Source: CAD feature listing. Evaluate the final solid. Frame: model axes, mm. A direction names the side the tool comes from. Round coordinates to 2 decimals unless told otherwise and drop trailing zeros.
Autodesk Fusion 360 part; units mm, degrees
sketch "Sketch1" plane through (0, 0, 0) normal (0, 1, 0) x (1, 0, 0)
  line L0 (20, -40) -> (-20, 40) construction
  line L1 (-20, -40) -> (20, 40) construction
  line L2 (5, 29) -> (-5, 29)
  line L3 (-5, 29) -> (-5, 39)
  line L4 (5, 39) -> (5, 29)
  line L5 (5, 29) -> (-5, 39) construction
  line L6 (-5, 29) -> (5, 39) construction
  line L7 (-4, 39) -> (-4, 40)
  line L8 (4, 39) -> (4, 40)
  line L9 (-19, 25) -> (-9, 25)
  line L10 (-9, 25) -> (-9, 15)
  line L11 (-9, 15) -> (-19, 15)
  line L12 (19, 25) -> (9, 25)
  line L13 (9, 25) -> (9, 15)
  line L14 (9, 15) -> (19, 15)
  line L15 (-20, 16) -> (-19, 16)
  line L16 (-19, 24) -> (-20, 24)
  line L17 (19, 16) -> (20, 16)
  line L18 (20, 24) -> (19, 24)
  line L19 (-20, 24) -> (-20, 40)
  line L20 (-19, 15) -> (-19, 16)
  line L21 (-19, 24) -> (-19, 25)
  line L22 (19, 15) -> (19, 16)
  line L23 (19, 24) -> (19, 25)
  line L24 (-20, 40) -> (-4, 40)
  line L25 (4, 40) -> (20, 40)
  line L26 (-5, 39) -> (-4, 39)
  line L27 (4, 39) -> (5, 39)
  line L28 (20, 40) -> (20, 24)
  line L29 (1.75, 0) -> (22.5, 0)
  line L30 (-19, -24) -> (-20, -24)
  line L31 (-19, -24) -> (-19, -25)
  line L32 (-19, -25) -> (-9, -25)
  line L33 (-20, -16) -> (-19, -16)
  line L34 (-19, -15) -> (-19, -16)
  line L35 (-9, -15) -> (-19, -15)
  line L36 (-9, -25) -> (-9, -15)
  line L37 (-4, -39) -> (-4, -40)
  line L38 (-5, -39) -> (-4, -39)
  line L39 (-5, -29) -> (-5, -39)
  line L40 (5, -29) -> (-5, -29)
  line L41 (5, -39) -> (5, -29)
  line L42 (4, -39) -> (5, -39)
  line L43 (4, -39) -> (4, -40)
  line L44 (20, -24) -> (19, -24)
  line L45 (19, -24) -> (19, -25)
  line L46 (19, -25) -> (9, -25)
  line L47 (9, -25) -> (9, -15)
  line L48 (9, -15) -> (19, -15)
  line L49 (19, -15) -> (19, -16)
  line L50 (19, -16) -> (20, -16)
  line L51 (-20, -40) -> (-20, -24)
  line L52 (-20, -16) -> (-20, 16)
  line L53 (20, 16) -> (20, -16)
  line L54 (20, -24) -> (20, -40)
  line L55 (20, -40) -> (4, -40)
  line L56 (-4, -40) -> (-20, -40)
  point P0 (0, 34)
  dimension "d20" = 40
  dimension "d21" = 80
  dimension "d22" = 10
  dimension "d23" = 10
  dimension "d24" = 20
  dimension "d25" = 16
  dimension "d26" = 16
  dimension "d27" = 1
  dimension "d28" = 15
  dimension "d29" = 15
  dimension "d30" = 10
  dimension "d31" = 10
  dimension "d32" = 10
  dimension "d33" = 10
  dimension "d34" = 16
  dimension "d35" = 8
  dimension "d36" = 1
  dimension "d37" = 16
  dimension "d38" = 8
  dimension "d39" = 1
extrude "Extrude1" add sketch "Sketch1" along normal blind 1300
sketch "Sketch2" plane through (20, 0, 0) normal (1, 0, 0) x (0, 1, 0)
  line L0 (0, 16) -> (0, -16)
  line L1 (0, -16) -> (1300, -16)
  line L2 (1300, -16) -> (1300, 16)
  line L3 (1300, 16) -> (0, 16)
  circle A0 centre (40, 0) radius 10
  circle A1 centre (1260, 0) radius 10
  dimension "d42" = 20
  dimension "d45" = 20
  dimension "d48" = 40
  dimension "d49" = 40
extrude "Extrude2" cut sketch "Sketch2" against normal blind 40 contours A0
extrude "Extrude3" cut sketch "Sketch2" against normal blind 35 contours A1
1. Line query: line 1 along Z through (x, y) = (15, 619); line 2 along Z through (x, y) = (11, 1260); line 3 along Z through (x, y) = (-7, 40). Output: solid intervals per line, ascending.
2. Pull-direction query (Z, two-part tool) for faces 3 (the face through (2.745, 1269.237, -3.83)), 4 (the face through (0, 30, 0)), 5 (the face through (0, 1300, -1)); classes: released by +Z, released by -Z, zero draft, split by the parting line, or undercut.
3. Access query for faces 1 (the face through (20, 641, 0)), 2 (the face through (-15, 1260, 0)). Directions: +Z, -Z, +X, -X, +Y, -Y. A direction counts if a zero-diameter tool reaches every point of the face in a straight line with its end or side. Return the directions, or none.
4. First-contact query: pin 1 (5 mm diameter, centred on y = 506, z = -21, fed in from -X); pin 2 (1.5 mm diameter, centred on y = 259, z = 22.5, fed in from +X); pin 3 (1.5 mm diameter, centred on x = 13, z = -10.5, fed in from -Y). Flat tips, straight axial feed; report the tip coordinate or a pass-through.
Result:
1. line 1: z = -40 to -25, -15 to 15, 25 to 40
1. line 2: z = -40 to -25, -15 to -10, 10 to 15, 25 to 40
1. line 3: z = -40 to -10, 10 to 40
2. face 3: undercut
2. face 4: undercut
2. face 5: zero draft
3. face 1: +Z, -Z, +X, +Y, -Y
3. face 2: +X
4. pin 1: stops at x = -9
4. pin 2: stops at x = 9
4. pin 3: stops at y = 0
